```python
from build123d import *

# Parameters (mm, degrees)
F2_R = 1.27
F3_R = 0.50799


# Not quite as in the source:
# - a fillet or chamfer is up to 0.001 mm smaller than in the source, because OpenCascade refuses the exact size


with BuildPart() as f1:
    # F0 (on Front) → F1 (revolve)
    with BuildSketch(Plane.XZ):
        with BuildLine():
            Line((-17.5, 0), (-6.604, 0))
            Line((-6.604, 0), (-6.604, 21.1916357695))
            Line((-6.604, 21.1916357695), (-8.9683642305, 21.1916357695))
            ThreePointArc((-8.9683642305, 21.1916357695), (-9.0925574741, 21.1401932437), (-9.144, 21.016))
            Line((-9.144, 21.016), (-9.144, 20.508))
            Line((-9.144, 20.508), (-10.414, 20.508))
            Line((-10.414, 20.508), (-10.414, 16.008))
            Line((-10.414, 16.008), (-9.144, 16.008))
            Line((-9.144, 16.008), (-9.144, 15.5))
            Line((-9.144, 15.5), (-7.874, 15.5))
            Line((-7.874, 15.5), (-7.874, 4))
            Line((-7.874, 4), (-16, 4))
            Line((-16, 4), (-16, 2))
            Line((-16, 2), (-17.5, 2))
            Line((-17.5, 2), (-17.5, 0))
        make_face()
    revolve(axis=Axis((0, 0, 10.5958178848), (0, 0, -1)))

    # F2
    f2_edges = [f1.edges().sort_by_distance(p)[0] for p in [
        (16, 0, 4),
        (17.5, 0, 2),
    ]]
    fillet(f2_edges, radius=F2_R)

    # F3 (radius 0.508 in the source; OpenCascade refuses exactly that, so slightly less here)
    f3_edges = [f1.edges().sort_by_distance(p)[0] for p in [
        (9.144, 0, 15.5),
    ]]
    fillet(f3_edges, radius=F3_R)


solid = f1.part
```
Read the model definition and answer for the solid it produces. Units are mm, in the model's axes. A direction names the side the tool comes from. Give positions to 0.01 mm unless a question says otherwise; leave off trailing zeros. Order: outer loops, then holes, each group sorted by start corner. A loop starts at its lowest first (then second) coordinate and runs counter-clockwise, first axis right, second up.
(1) Find section A-A (z = 20). Give the vertices of the cut face in (x, y).
(2) Find section B-B (z = 5.25). Give the vertices of the cut face in (x, y), plus the area to 3 significant figures.
(3) Straight lines are drawn through the part: L1, parallel to Y at x = 0, z = 8; L2, parallel to Z at x = -3.5, y = 7.5; L3, parallel to Z at x = -1, y = -11.5. For each, find the intervals that lie inside material, in ascending order.
(4) For faces 4 (the flat face through (6, -6, 4)), 5 (the cylindrical face through (13.887, -10.648, 0.36)), 6 (the flat face through (5, -8, 20.508)), determine the directions among +Z, -Z, +X, -X, +Y, -Y from which every point of the face is accessible in a straight line to the end or side of a thin tool.
(5) For a pull along Z with two mould halves and no side action, classify faces 1 (the flat face through (-8, 2, 15.5)), 2 (the cylindrical face through (-6.1, -2.53, 10.74)), 3 (the flat face through (0, -8, 0)) as released by +Z, released by -Z, zero draft, split by the parting line, or undercut.
(6) Given pin 1 (2 mm diameter, centred on x = 0, y = -4, fed in from +Z); pin 2 (5 mm diameter, centred on x = 1.5, z = 10, fed in from -Y); pin 3 (1 mm diameter, centred on x = 4.5, z = 12.5, fed in from +Y); pin 4 (12 mm diameter, centred on y = -3.5, z = 9, fed in from +X), each flat-ended and moving along its own axis, determine where each tip first touches the part or whether it passes through.
Result sheet:
1. outline: circle Ø20.83 at (0, 0); hole circle Ø13.21 at (0, 0)
2. outline: circle Ø15.75 at (0, 0); hole circle Ø13.21 at (0, 0)
2. area: 57.8 mm2
3. L1: y = -7.87 to -6.6, 6.6 to 7.87
3. L2: z = 0 to 4, 15.5 to 21.19
3. L3: z = 0 to 4
4. face 4: none
4. face 5: +Z, -Z
4. face 6: +Z
5. face 1: undercut
5. face 2: zero draft
5. face 3: released by -Z
6. pin 1: passes through
6. pin 2: stops at y = -7.87
6. pin 3: stops at y = 6.78
6. pin 4: stops at x = 15.79
